```python
from build123d import *

# Parameters (mm, degrees)
F4_DEPTH  = 19.5
F5_DEPTH  = 4
F6_DEPTH  = 11.5
F7_DEPTH  = 8.5
F9_COUNT  = 3
F9_ANGLE  = 240
F2_R      = 1.75
F2_R_2    = 6
F10_DEPTH = 4
F11_R     = 6.5
F12_DEPTH = 20
F13_DEPTH = 4


# Not quite as in the source:
# - a feature of the source that left no trace in its solid (it failed there, or was rolled back) is left out
# - a feature names something its author has since deleted; it is built from what else it names


with BuildPart() as f3:
    # F0 (on Top) → F3 (revolve)
    with BuildSketch(Plane.XY):
        Polygon((19.5, 34), (0, 34), (0, 31.7), (22.5, 31.7), (22.5, 32.7), align=None)
    revolve(axis=Axis((11.25, 30, 0), (1, 0, 0)))

    # F1 (on Right) → F4 (join)
    with BuildSketch(Plane.YZ):
        with BuildLine():
            Line((26, 4), (26, 0))
            ThreePointArc((26, 0), (27.1715728753, 2.8284271247), (30, 4))
            Line((30, 4), (26, 4))
        make_face()
        with BuildLine():
            Line((26, -4), (30, -4))
            ThreePointArc((30, -4), (27.1715728753, -2.8284271247), (26, 0))
            Line((26, 0), (26, -4))
        make_face()
    extrude(amount=F4_DEPTH)

    # F0 (on Top) → F5 (join, symmetric)
    with BuildSketch(Plane.XY):
        Polygon((19.5, 26), (0, 26), (0, 0), (25.8833302492, 14.9437476869), align=None)
    extrude(amount=F5_DEPTH, both=True)

    # F1 (on Right) → F6 (cut)
    with BuildSketch(Plane.YZ):
        Polygon((30, -3.4063665882), (32.95, -1.7031832941), (32.95, 1.7031832941), (30, 3.4063665882), (27.05, 1.7031832941), (27.05, -1.7031832941), align=None)
    extrude(amount=F6_DEPTH, mode=Mode.SUBTRACT)

    # F1 (on Right) → F7 (cut)
    with BuildSketch(Plane.YZ):
        with BuildLine():
            Line((32.95, 1.7031832941), (32.95, -1.7031832941))
            Line((32.95, -1.7031832941), (30, -3.4063665882))
            Line((30, -3.4063665882), (30, -4))
            ThreePointArc((30, -4), (32.8284271247, -2.8284271247), (34, 0))
            ThreePointArc((34, 0), (32.8284271247, 2.8284271247), (30, 4))
            Line((30, 4), (30, 3.4063665882))
            Line((30, 3.4063665882), (32.95, 1.7031832941))
        make_face()
    extrude(amount=F7_DEPTH, mode=Mode.SUBTRACT)

    # F8: F3 across plane


with BuildPart() as f3_1:
    add(f3.part)
    add(f3.part.mirror(Plane.YZ))

    # F9: F3 ×3 about axis
    f9_axis = Axis((0, 0, 0), (0, 0, -1))


with BuildPart() as f3_2:
    add(f3_1.part)
    for i in range(1, F9_COUNT):
        add(f3_1.part.rotate(f9_axis, i * F9_ANGLE / (F9_COUNT - 1)))

    # F2 (on Top) → F10 (cut, symmetric)
    with BuildSketch(Plane.XY):
        with Locations((14.5, 17)):
            Circle(F2_R)
        with BuildLine():
            add(Edge.make_bspline(
                [(12.5257586532, 14.3151527465), (13.3123168346, 13.9246002449), (14.4418337404, 12.6938657), (14.9288469383, 11.0046443666), (15, 10)],
                knots=[0, 0, 0, 0, 0.4852212686, 1, 1, 1, 1], degree=3))
            Line((12.5257586532, 14.3151527465), (2.4642293228, 16.8734356371))
            ThreePointArc((2.4642293228, 16.8734356371), (0, 17.1818117358), (-2.4642293228, 16.8734356371))
            Line((-2.4642293228, 16.8734356371), (-12.5257586532, 14.3151527465))
            add(Edge.make_bspline(
                [(-12.5257586532, 14.3151527465), (-13.3123168346, 13.9246002449), (-14.4418337404, 12.6938657), (-14.9288469383, 11.0046443666), (-15, 10)],
                knots=[0, 0, 0, 0, 0.4852212686, 1, 1, 1, 1], degree=3))
            Line((-15, 10), (-15, 0))
            Line((-15, 0), (-15, -10))
            add(Edge.make_bspline(
                [(-12.5257586532, -14.3151527465), (-13.3123168346, -13.9246002449), (-14.4418337404, -12.6938657), (-14.9288469383, -11.0046443666), (-15, -10)],
                knots=[0, 0, 0, 0, 0.4852212686, 1, 1, 1, 1], degree=3))
            Line((-12.5257586532, -14.3151527465), (-2.4642293228, -16.8734356371))
            ThreePointArc((-2.4642293228, -16.8734356371), (0, -17.1818117358), (2.4642293228, -16.8734356371))
            Line((2.4642293228, -16.8734356371), (12.5257586532, -14.3151527465))
            add(Edge.make_bspline(
                [(12.5257586532, -14.3151527465), (13.3123168346, -13.9246002449), (14.4418337404, -12.6938657), (14.9288469383, -11.0046443666), (15, -10)],
                knots=[0, 0, 0, 0, 0.4852212686, 1, 1, 1, 1], degree=3))
            Line((15, -10), (15, 0))
            Line((15, 0), (15, 10))
        make_face()
        with Locations((-14.5, 17)):
            Circle(F2_R)
        with Locations((-14.5, -17)):
            Circle(F2_R)
        with Locations((14.5, -17)):
            Circle(F2_R)
        with Locations((-24, 0)):
            Circle(F2_R_2)
        with Locations((24, 0)):
            Circle(F2_R_2)
    extrude(amount=F10_DEPTH, both=True, mode=Mode.SUBTRACT)

    # F11 (on Top) → F12 (cut, symmetric)
    with BuildSketch(Plane.XY):
        Polygon((4.9074772881, -21.4), (-4.9074772881, -21.4), (-9.8149545762, -29.9), (-4.9074772881, -38.4), (4.9074772881, -38.4), (9.8149545762, -29.9), align=None)
        with Locations((0, -29.9)):
            Circle(F11_R, mode=Mode.SUBTRACT)
        with Locations((0, -29.9)):
            Circle(F11_R)
    extrude(amount=F12_DEPTH, both=True, mode=Mode.SUBTRACT)

    # F11 (on Top) → F13 (join)
    with BuildSketch(Plane.XY):
        Polygon((4.9074772881, -21.4), (-4.9074772881, -21.4), (-9.8149545762, -29.9), (-4.9074772881, -38.4), (4.9074772881, -38.4), (9.8149545762, -29.9), align=None)
        with Locations((0, -29.9)):
            Circle(F11_R, mode=Mode.SUBTRACT)
    extrude(amount=-F13_DEPTH)


solid = f3_2.part
```
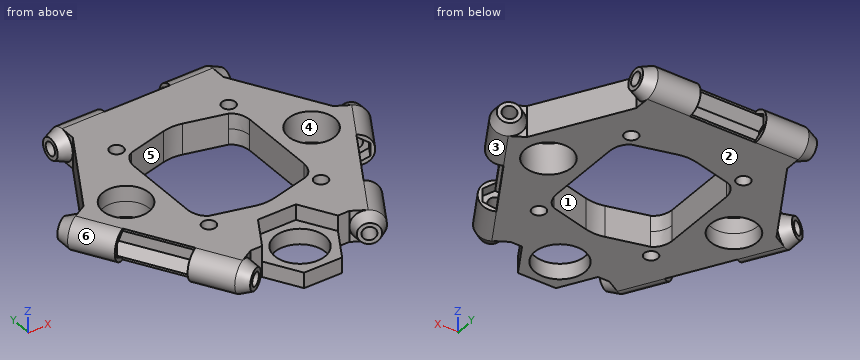
Here's how the part is built. I have some questions about the finished solid (model axes, mm). Face numbers are marked on the shaded views. A direction names the side the tool comes from. Coordinates: 2 decimals unless noted, no trailing zeros. Order: outer loops, then holes, each group sorted by start corner. A loop starts at its lowest first (then second) coordinate and runs counter-clockwise, first axis right, second up. Notation, with made-up numbers: (16, 71.25) -> (34, 71.25) arc R17 ccw to (34, 86.25) -> close; hole circle Ø7 at (-23.75, 21.25). An arc over 180 degrees is marked (long way). Return JSON: item names as keys, results as strings.
1) If I drill on probe 1 along Y at (x, z) = (6, -2); probe 2 along Y at (x, z) = (-12, -0.75); probe 3 along Y at (x, z) = (14, -3.5), over which ranges is the centre line in solid material (lowest first)?
Conclusion:
{"probe 1": "y = -36.51 to -32.4, -27.4 to -15.97, 15.97 to 27.56", "probe 2": "y = -29.89 to -14.45, 14.45 to 28.47, 31.53 to 33.93", "probe 3": "y = -30.6 to -18.68, -15.32 to -13.03, 13.03 to 15.32, 18.68 to 31.94"}
2) On a 3-axis mill with a long thin cutter (end or side, diameter ignored), from which of +Z, -Z, +X, -X, +Y, -Y can I reach the whole of each face in a straight line? I mean the marked faces 1 and 2. Say none if no direction works.
Conclusion:
{"face 1": "+Z, -Z", "face 2": "-Z, +X, -X, +Y, -Y"}
3) If we section it at A-A on x = 0: List the corners of the cut face in (y, z) for me, plus the area to 3 significant figures.
Conclusion:
{"outline": "(-38.4, -4) -> (-36.4, -4) -> (-36.4, 0) -> (-38.4, 0) -> close; (-23.4, -4) -> (-17.18, -4) -> (-17.18, 4) -> (-21.4, 4) -> (-21.4, 0) -> (-23.4, 0) -> close; (17.18, -4) -> (30, -4) -> (30, -3.41) -> (27.05, -1.7) -> (27.05, 1.7) -> (30, 3.41) -> (30, 4) -> (17.18, 4) -> close", "area": "137 mm²"}
4) If we section it at B-B on y = 8.5: List the corners of the cut face in (x, z) for me.
Conclusion:
{"outline": "(-29.6, -4) -> (-15, -4) -> (-15, 4) -> (-29.6, 4) -> close; (15, -4) -> (29.6, -4) -> (29.6, 4) -> (15, 4) -> close"}
5) Thinking about a two-plate mould opening in X: for the marked faces 3, 4, 5 and 6, which applies, +X half, -X half, draft (parallel to the pull), parting line (faces both ways), or undercut?
Conclusion:
{"face 3": "+X half", "face 4": "undercut", "face 5": "undercut", "face 6": "-X half"}
6) If we section it at C-C on y = -27.5: State how many separate pieces and enclosed holes the cut face has, plus the area to 3 significant figures.
Conclusion:
{"separate pieces": "2", "enclosed holes": "2", "area": "222 mm²"}
7) I'm going to push flat-ended pins straight in: P1, Ø2.5, axis at x = 9.5, z = -0.5, coming from the -Y side; P2, Ø2, axis at y = 7, z = -3, coming from the -X side; P3, Ø5, axis at x = -1.5, y = -32, coming from the +Z side; P4, Ø1.5, axis at x = -10.5, z = -0.5, coming from the -Y side. Where does each tip first touch, or does it pass through?
Conclusion:
{"P1": "stops at y = -32.61", "P2": "stops at x = -31.05", "P3": "passes through", "P4": "stops at y = -30.01"}
